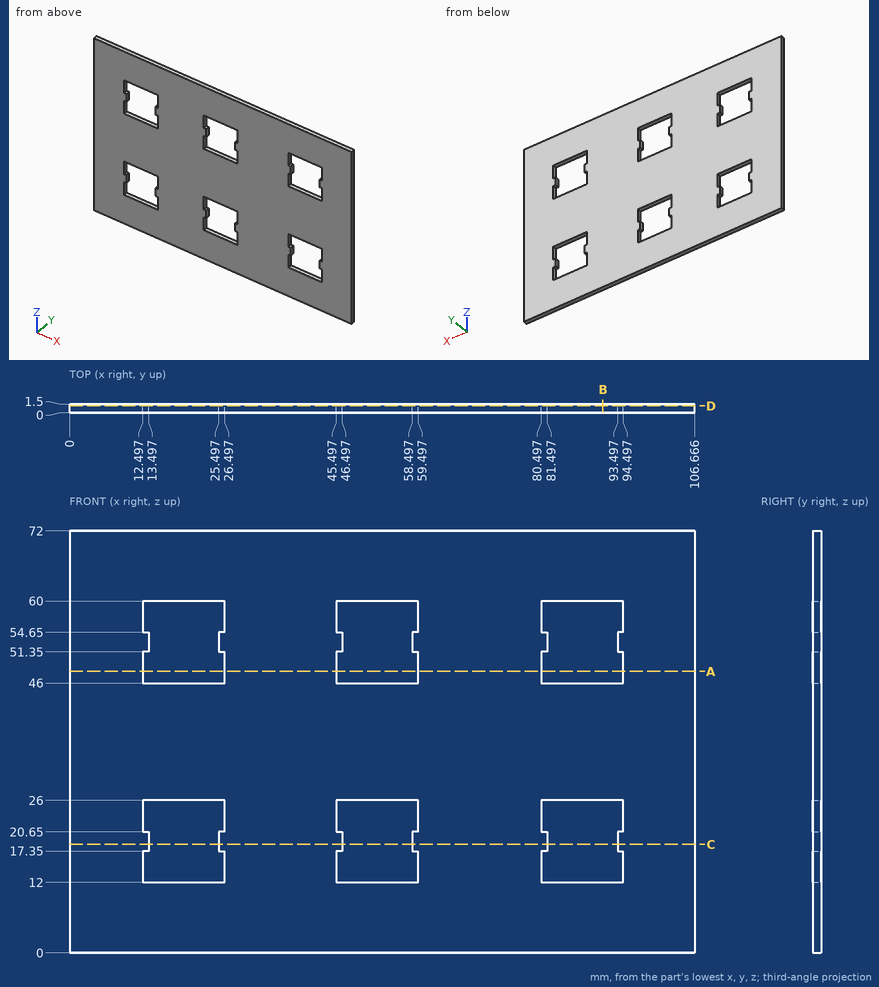
Verification items for this drawing (mm, ordinates from the low corner). Round coordinates to 2 decimals unless told otherwise and drop trailing zeros. Write each loop counter-clockwise with the first axis right and the second up, starting at its lowest first coordinate (ties: lowest second). Pieces come first, ordered by that corner, then holes. Notation, with made-up numbers: (36.5, -36) - (66.5, -36) arc R22 ccw to (66.5, -17) - close; hole circle Ø4 at (15.5, 48.5). An arc over 180 degrees is marked (long way). One line per item, written item: value.
1. Cross-section at A-A on z = 48. Record the boundary of the cut face in (x, y) (1 decimal).
The answers:
outline: (0, 0) - (12.5, 0) - (12.5, 1.5) - (0, 1.5) - close; (26.5, 0) - (45.5, 0) - (45.5, 1.5) - (26.5, 1.5) - close; (59.5, 0) - (80.5, 0) - (80.5, 1.5) - (59.5, 1.5) - close; (94.5, 0) - (106.7, 0) - (106.7, 1.5) - (94.5, 1.5) - close
2. Scan lines: L1, parallel to X at y = 0.3, z = 50 (1 decimal); L2, parallel to Z at x = 23.5, y = 0.8; L3, parallel to X at y = 0.95, z = 18.5 (1 decimal). Record each from-to range of solid material in increasing order.
The answers:
L1: x = 0 to 12.5, 26.5 to 45.5, 59.5 to 80.5, 94.5 to 106.7
L2: z = 0 to 12, 26 to 46, 60 to 72
L3: x = 0 to 13.5, 25.5 to 46.5, 58.5 to 81.5, 93.5 to 106.7
3. Cross-section at D-D on y = 1.2. Give the number of separate pieces and of enclosed holes in the cut face, and give its area (3 significant figures).
The answers:
separate pieces: 1
enclosed holes: 6
area: 6,540 mm^2
4. Cross-section at B-B on x = 91. Record the boundary of the cut face in (y, z).
The answers:
outline: (0, 0) - (1.5, 0) - (1.5, 12) - (0, 12) - close; (0, 26) - (1.5, 26) - (1.5, 46) - (0, 46) - close; (0, 60) - (1.5, 60) - (1.5, 72) - (0, 72) - close
5. Cross-section at C-C on z = 18.5. Record the boundary of the cut face in (x, y) (1 decimal).
The answers:
outline: (0, 0) - (13.5, 0) - (13.5, 1.5) - (0, 1.5) - close; (25.5, 0) - (46.5, 0) - (46.5, 1.5) - (25.5, 1.5) - close; (58.5, 0) - (81.5, 0) - (81.5, 1.5) - (58.5, 1.5) - close; (93.5, 0) - (106.7, 0) - (106.7, 1.5) - (93.5, 1.5) - close
